```python
from build123d import *

# Parameters (mm, degrees)
SKETCH1_R           = 2.0999999
BOSS_EXTRUDE2_DEPTH = 400


# Read off the part's stored shape, not the designer's step: Imported1
with BuildPart() as part:
    # Sketch1 → Boss-Extrude2 (new body)
    with BuildSketch(Plane.XY.offset(10)):
        with BuildLine():
            Line((15.999999496, 12), (12.9999995, 12))
            Line((12.9999995, 12), (12.9999995, 10.3))
            ThreePointArc((12.9999995, 10.3), (13.087867466, 10.087867966), (13.2999995, 10))
            Line((13.2999995, 10), (26.7, 10))
            ThreePointArc((26.7, 10), (26.912132034, 10.087867966), (27, 10.3))
            Line((27, 10.3), (27, 12))
            Line((27, 12), (24, 12))
            Line((24, 12), (24, 12.9393436))
            Line((24, 12.9393436), (27.06068075, 16))
            Line((27.06068075, 16), (29.480384758, 16))
            Line((29.480384758, 16), (30, 16.3))
            Line((30, 16.3), (30.519615242, 16))
            Line((30.519615242, 16), (32.93933675, 16))
            Line((32.93933675, 16), (36, 12.9393398))
            Line((36, 12.9393398), (36, 12))
            Line((36, 12), (33, 12))
            Line((33, 12), (33, 10.3))
            ThreePointArc((33, 10.3), (33.087867966, 10.087867966), (33.3, 10))
            Line((33.3, 10), (39, 10))
            ThreePointArc((39, 10), (39.707106781, 10.292893219), (40, 11))
            Line((40, 11), (40, 16.7))
            ThreePointArc((40, 16.7), (39.912132034, 16.912132034), (39.7, 17))
            Line((39.7, 17), (38, 17))
            Line((38, 17), (38, 14))
            Line((38, 14), (37.0606655, 13.99999425))
            Line((37.0606655, 13.99999425), (34, 17.060646))
            Line((34, 17.060646), (34, 19.480361375))
            Line((34, 19.480361375), (33.6999865, 20))
            Line((33.6999865, 20), (33.9999865, 20.519615242))
            Line((33.9999865, 20.519615242), (33.9999865, 22.9393395))
            Line((33.9999865, 22.9393395), (37.060675, 25.999997))
            Line((37.060675, 25.999997), (38, 25.999997))
            Line((38, 25.999997), (38, 23))
            Line((38, 23), (39.7, 23))
            ThreePointArc((39.7, 23), (39.912132034, 23.087867966), (40, 23.3))
            Line((40, 23.3), (40, 29))
            ThreePointArc((40, 29), (39.707106781, 29.707106781), (39, 30))
            Line((39, 30), (33.3, 30))
            ThreePointArc((33.3, 30), (33.087867966, 29.912132034), (33, 29.7))
            Line((33, 29.7), (33, 28))
            Line((33, 28), (36, 28))
            Line((36, 28), (36, 27.0606575))
            Line((36, 27.0606575), (32.9393565, 24))
            Line((32.9393565, 24), (30.519615242, 24))
            Line((30.519615242, 24), (30, 23.7))
            Line((30, 23.7), (29.480384758, 24))
            Line((29.480384758, 24), (27.06066, 24))
            Line((27.06066, 24), (24.0000025, 27.0606565))
            Line((24.0000025, 27.0606565), (24.0000025, 28))
            Line((24.0000025, 28), (27, 28))
            Line((27, 28), (27, 29.7))
            ThreePointArc((27, 29.7), (26.912132034, 29.912132034), (26.7, 30))
            Line((26.7, 30), (13.2999995, 30))
            ThreePointArc((13.2999995, 30), (13.087867466, 29.912132034), (12.9999995, 29.7))
            Line((12.9999995, 29.7), (12.9999995, 28))
            Line((12.9999995, 28), (15.9999995, 28))
            Line((15.9999995, 28), (15.9999995, 27.06066257))
            Line((15.9999995, 27.06066257), (12.9393312, 24))
            Line((12.9393312, 24), (10.519614742, 24))
            Line((10.519614742, 24), (9.9999995, 23.7))
            Line((9.9999995, 23.7), (9.480384258, 24))
            Line((9.480384258, 24), (7.0606425, 24))
            Line((7.0606425, 24), (3.9999995, 27.0606365))
            Line((3.9999995, 27.0606365), (3.9999995, 28))
            Line((3.9999995, 28), (6.9999995, 28))
            Line((6.9999995, 28), (6.9999995, 29.7))
            ThreePointArc((6.9999995, 29.7), (6.912131534, 29.912132034), (6.6999995, 30))
            Line((6.6999995, 30), (1, 30))
            ThreePointArc((1, 30), (0.292893219, 29.707106781), (0, 29))
            Line((0, 29), (0, 23.3))
            ThreePointArc((0, 23.3), (0.087867966, 23.087867966), (0.3, 23))
            Line((0.3, 23), (2, 23))
            Line((2, 23), (2, 25.999998))
            Line((2, 25.999998), (2.9393195, 25.999998))
            Line((2.9393195, 25.999998), (6, 22.939318))
            Line((6, 22.939318), (6, 20.519615242))
            Line((6, 20.519615242), (6.3, 20))
            Line((6.3, 20), (6, 19.480384758))
            Line((6, 19.480384758), (6, 17.0606635))
            Line((6, 17.0606635), (2.9393372, 14))
            Line((2.9393372, 14), (2, 14))
            Line((2, 14), (2, 17))
            Line((2, 17), (0.3, 17))
            ThreePointArc((0.3, 17), (0.087867966, 16.912132034), (0, 16.7))
            Line((0, 16.7), (0, 11))
            ThreePointArc((0, 11), (0.292893219, 10.292893219), (1, 10))
            Line((1, 10), (6.6999995, 10))
            ThreePointArc((6.6999995, 10), (6.912131534, 10.087867966), (6.9999995, 10.3))
            Line((6.9999995, 10.3), (6.9999995, 12))
            Line((6.9999995, 12), (3.999991, 12))
            Line((3.999991, 12), (3.999991, 12.93933465))
            Line((3.999991, 12.93933465), (7.0606385, 16))
            Line((7.0606385, 16), (9.480384258, 16))
            Line((9.480384258, 16), (9.9999995, 16.3))
            Line((9.9999995, 16.3), (10.519614742, 16))
            Line((10.519614742, 16), (12.93931635, 16))
            Line((12.93931635, 16), (15.999999496, 12.9393436))
            Line((15.999999496, 12.9393436), (15.999999496, 12))
        make_face()
        with Locations(Location((9.9999995, 20, 0), (0, 0, 180))):
            Circle(SKETCH1_R, mode=Mode.SUBTRACT)
        with Locations(Location((30, 20, 0), (0, 0, 180))):
            Circle(SKETCH1_R, mode=Mode.SUBTRACT)
        with BuildLine():
            Line((17.99999975, 12.936400074), (17.99999975, 12.3))
            ThreePointArc((17.99999975, 12.3), (18.087867716, 12.087867966), (18.29999975, 12))
            Line((18.29999975, 12), (21.6999995, 12))
            ThreePointArc((21.6999995, 12), (21.912131534, 12.087867966), (21.9999995, 12.3))
            Line((21.9999995, 12.3), (21.9999995, 12.936400498))
            ThreePointArc((21.9999995, 12.936400498), (22.022835631, 13.051205559), (22.087867469, 13.148532591))
            Line((22.087867469, 13.148532591), (26, 17.0606645))
            Line((26, 17.0606645), (26, 22.939339))
            Line((26, 22.939339), (22.087867469, 26.851468459))
            ThreePointArc((22.087867469, 26.851468459), (22.022835646, 26.948794955), (21.9999995, 27.063599552))
            Line((21.9999995, 27.063599552), (21.9999995, 27.7))
            ThreePointArc((21.9999995, 27.7), (21.912131534, 27.912132034), (21.6999995, 28))
            Line((21.6999995, 28), (18.29999975, 28))
            ThreePointArc((18.29999975, 28), (18.087867716, 27.912132034), (17.99999975, 27.7))
            Line((17.99999975, 27.7), (17.99999975, 27.063604538))
            ThreePointArc((17.99999975, 27.063604538), (17.977163602, 26.948799949), (17.912131781, 26.851473459))
            Line((17.912131781, 26.851473459), (14, 22.939335))
            Line((14, 22.939335), (14, 17.06066805))
            Line((14, 17.06066805), (17.912135369, 13.14852345))
            ThreePointArc((17.912135369, 13.14852345), (17.977164541, 13.051200418), (17.99999975, 12.936400074))
        make_face(mode=Mode.SUBTRACT)
    extrude(amount=-BOSS_EXTRUDE2_DEPTH)


solid = part.part
```
Here's how the part is built. I have some questions about the finished solid (model axes, mm). Round coordinates to 2 decimals unless told otherwise and drop trailing zeros. Answer in a Markdown table with one row per item.
Item 1: I'm going to push flat-ended pins straight in: pin 1 (1 mm diameter, centred on y = 21.5, z = -335, fed in from +X); pin 2 (1.2 mm diameter, centred on x = 8, z = -145.5, fed in from +Y); pin 3 (2 mm diameter, centred on x = 28.5, z = -112.5, fed in from -Y). Where does each tip first touch, or does it pass through?
A:
| item | result |
|---|---|
| pin 1 | stops at x = 34 |
| pin 2 | stops at y = 24 |
| pin 3 | stops at y = 16 |
Item 2: Imagine slicing it at A-A, the plane z = -111.5. State how many separate pieces and enclosed holes the cut face has, and give its area (3 significant figures).
A:
| item | result |
|---|---|
| separate pieces | 1 |
| enclosed holes | 3 |
| area | 324 mm2 |
Item 3: If I drill on L1, parallel to X at y = 20, z = -83; L2, parallel to X at y = 13, z = -304; L3, parallel to X at y = 11, z = -321.5, over which ranges is the centre line in solid material (lowest first)? Write a range as from..to.
A:
| item | result |
|---|---|
| L1 | x = 6.3..7.9, 12.1..14, 26..27.9, 32.1..33.7 |
| L2 | x = 0..4.06, 15.94..17.99, 22.01..24.06, 35.94..40 |
| L3 | x = 0..7, 13..27, 33..40 |
